from build123d import *

# Parameters (mm, degrees)
SKETCH001_AS_DRAWN_R                 = 9.6
EXTRUDE001_DEPTH                     = 6
EXTRUDE001_ONTO_SKETCH001_ROLL_ANGLE = 90
SKETCH_AS_DRAWN_W                    = 75
SKETCH_AS_DRAWN_H                    = 83
SKETCH_AS_DRAWN_R                    = 5.5
EXTRUDE_DEPTH                        = 10
EXTRUDE_ONTO_SKETCH_ROLL_ANGLE       = 90


with BuildPart() as obj1:
    # Sketch001 as drawn → Extrude001 (new)
    with BuildSketch(Plane.XY):
        Circle(SKETCH001_AS_DRAWN_R)
    extrude(amount=-EXTRUDE001_DEPTH)


with BuildPart() as obj1_1:
    # Extrude001 onto Sketch001 roll: moved
    add(obj1.part.rotate(Axis((0, 0, 0), (1, 0, 0)), EXTRUDE001_ONTO_SKETCH001_ROLL_ANGLE))


with BuildPart() as obj1_2:
    # Extrude001 onto Sketch001 placement: moved
    add(obj1_1.part)


with BuildPart() as obj2:
    # Sketch as drawn → Extrude (new)
    with BuildSketch(Plane.XY):
        with Locations((0, 23.5)):
            Rectangle(SKETCH_AS_DRAWN_W, SKETCH_AS_DRAWN_H)
        Circle(SKETCH_AS_DRAWN_R, mode=Mode.SUBTRACT)
    extrude(amount=-EXTRUDE_DEPTH)


with BuildPart() as obj2_1:
    # Extrude onto Sketch roll: moved
    add(obj2.part.rotate(Axis((0, 0, 0), (1, 0, 0)), EXTRUDE_ONTO_SKETCH_ROLL_ANGLE))


with BuildPart() as obj2_2:
    # Extrude onto Sketch placement: moved
    add(obj2_1.part)

    # Cut: cut obj1
    add(obj1_2.part, mode=Mode.SUBTRACT)


solid = obj2_2.part
Verification items for the finished model (mm, model axes). A direction names the side the tool comes from. Give positions to 0.01 mm unless a question says otherwise; leave off trailing zeros. Loops run counter-clockwise (first coordinate to the right, second up) from the corner with the lowest first, then second, coordinate; pieces in that order, holes last. Notation, with made-up numbers: (56, -1.5) - (94, -1.5) arc R27 ccw to (94, 21.5) - close; hole circle Ø1 at (-36, 67). An arc over 180 degrees is marked (long way). Write item = value, one per line. Start each with the question number.
Q1. Thickness scan on line 1 (Z direction, x = 0, y = 2); line 2 (Z direction, x = 0, y = 7.6); line 3 (X direction, y = 5.25, z = 8). Record the ranges inside material, lowest first.
Q2. Cross-section at D-D, the plane y = 3.5. Enter the section's corners in (x, z).
Q3. Mould release check, pull along Z, two halves, no side actions. Record for faces 3 (the face through (-1, 5, -18)), 4 (the face through (-1, 5, 65)), 5 (the face through (5.161, 2.958, 8.095)), 6 (the face through (-37.5, 5, 23)): released by +Z, released by -Z, zero draft, split by the parting line, or undercut.
Q4. Cross-section at A-A, the plane x = 0. Enter the section's corners in (y, z), and give its area (3 significant figures).
Q5. Cross-section at C-C, the plane y = 9. Enter the section's corners in (x, z), and give its area (3 significant figures).
Q6. Tool access check on faces 1 (the face through (4, 6, -4)), 2 (the face through (37.5, 5, 23)). Record the directions out of +Z, -Z, +X, -X, +Y, -Y that give a thin tool (end or side, any length) a straight path to the whole face; none if there is none.
Q7. Cross-section at B-B, the plane z = 0. Enter the section's corners in (x, y).
Q8. Depth check by flat-ended pin: P1, Ø6.5, axis at x = 0, z = 0, coming from the +Y side; P2, Ø25, axis at x = 0, z = 0, coming from the -Y side. Enter the tip coordinate at first touch or a pass-through.
Answer key:
q1.line_1 = -18 to -9.6, 9.6 to 65
q1.line_2 = -18 to -5.5, 5.5 to 65
q1.line_3 = -37.5 to -5.31, 5.31 to 37.5
q2.outline = (-37.5, -18) - (37.5, -18) - (37.5, 65) - (-37.5, 65) - close; hole circle Ø19.2 at (0, 0)
q3.face_3 = released by -Z
q3.face_4 = released by +Z
q3.face_5 = undercut
q3.face_6 = zero draft
q4.outline = (0, -18) - (10, -18) - (10, -5.5) - (6, -5.5) - (6, -9.6) - (0, -9.6) - close; (0, 9.6) - (6, 9.6) - (6, 5.5) - (10, 5.5) - (10, 65) - (0, 65) - close
q4.area = 671 mm^2
q5.outline = (-37.5, -18) - (37.5, -18) - (37.5, 65) - (-37.5, 65) - close; hole circle Ø11 at (0, 0)
q5.area = 6,130 mm^2
q6.face_1 = -Y
q6.face_2 = +Z, -Z, +X, +Y, -Y
q7.outline = (-37.5, 0) - (-9.6, 0) - (-9.6, 6) - (-5.5, 6) - (-5.5, 10) - (-37.5, 10) - close; (5.5, 6) - (9.6, 6) - (9.6, 0) - (37.5, 0) - (37.5, 10) - (5.5, 10) - close
q8.P1 = through
q8.P2 = 0
